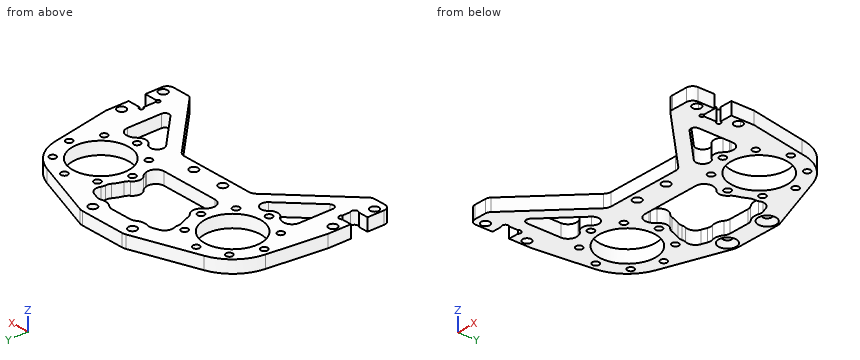
```python
from build123d import *

# Parameters (mm, degrees)
SKETCH_1_R          = 2.025
SKETCH_1_R_2        = 13.4
SKETCH_1_R_3        = 1.6
EXTRUDE_1_DEPTH     = 6
CHAMFER_1_SIZE      = 2.2
SKETCH_2_R          = 2.05
EXTRUDE_1_2_DEPTH   = 6
CUT_EXTRUDE_2_DEPTH = 7
SKETCH_4_R          = 1.525
CUT_EXTRUDE_3_DEPTH = 7
FILLET_1_R          = 3
CUT_EXTRUDE_6_DEPTH = 7
SKETCH_10_R         = 2.05
EXTRUDE_2_DEPTH     = 6
SKETCH_11_R         = 2.05
SKETCH_11_R_2       = 1
CUT_EXTRUDE_8_DEPTH = 7


with BuildPart() as part:
    # 草图1 → Extrude 1 (new body)
    with BuildSketch(Plane.XY):
        with BuildLine():
            Line((-43.507889071, -19.796198897), (-12.668545017, -30.71338069))
            ThreePointArc((-12.668545017, -30.71338069), (-11.846491746, -30.927824238), (-11, -31))
            Line((-11, -31), (11, -31))
            ThreePointArc((11, -31), (11.846491746, -30.927824238), (12.668545017, -30.71338069))
            Line((12.668545017, -30.71338069), (43.507889071, -19.796198897))
            ThreePointArc((43.507889071, -19.796198897), (57.5, 0), (43.507889071, 19.796198897))
            Line((43.507889071, 19.796198897), (12.668545017, 30.71338069))
            ThreePointArc((12.668545017, 30.71338069), (11.846491746, 30.927824238), (11, 31))
            Line((11, 31), (-11, 31))
            ThreePointArc((-11, 31), (-11.846491746, 30.927824238), (-12.668545017, 30.71338069))
            Line((-12.668545017, 30.71338069), (-43.507889071, 19.796198897))
            ThreePointArc((-43.507889071, 19.796198897), (-57.5, 0), (-43.507889071, -19.796198897))
        make_face()
        with Locations((-11, 26)):
            Circle(SKETCH_1_R, mode=Mode.SUBTRACT)
        with Locations((11, 26)):
            Circle(SKETCH_1_R, mode=Mode.SUBTRACT)
        with Locations((-36.5, 0)):
            Circle(SKETCH_1_R_2, mode=Mode.SUBTRACT)
        with Locations((-19, 0)):
            Circle(SKETCH_1_R_3, mode=Mode.SUBTRACT)
        with Locations((-24.125631329, -12.374368671)):
            Circle(SKETCH_1_R_3, mode=Mode.SUBTRACT)
        with Locations((-36.5, -17.5)):
            Circle(SKETCH_1_R_3, mode=Mode.SUBTRACT)
        with Locations((-48.874368671, -12.374368671)):
            Circle(SKETCH_1_R_3, mode=Mode.SUBTRACT)
        with Locations((-54, 0)):
            Circle(SKETCH_1_R_3, mode=Mode.SUBTRACT)
        with Locations((-48.874368671, 12.374368671)):
            Circle(SKETCH_1_R_3, mode=Mode.SUBTRACT)
        with Locations((-36.5, 17.5)):
            Circle(SKETCH_1_R_3, mode=Mode.SUBTRACT)
        with Locations((-24.125631329, 12.374368671)):
            Circle(SKETCH_1_R_3, mode=Mode.SUBTRACT)
        with Locations((36.5, 0)):
            Circle(SKETCH_1_R_2, mode=Mode.SUBTRACT)
        with Locations((19, 0)):
            Circle(SKETCH_1_R_3, mode=Mode.SUBTRACT)
        with Locations((24.125631329, 12.374368671)):
            Circle(SKETCH_1_R_3, mode=Mode.SUBTRACT)
        with Locations((36.5, 17.5)):
            Circle(SKETCH_1_R_3, mode=Mode.SUBTRACT)
        with Locations((48.874368671, 12.374368671)):
            Circle(SKETCH_1_R_3, mode=Mode.SUBTRACT)
        with Locations((54, 0)):
            Circle(SKETCH_1_R_3, mode=Mode.SUBTRACT)
        with Locations((48.874368671, -12.374368671)):
            Circle(SKETCH_1_R_3, mode=Mode.SUBTRACT)
        with Locations((36.5, -17.5)):
            Circle(SKETCH_1_R_3, mode=Mode.SUBTRACT)
        with Locations((24.125631329, -12.374368671)):
            Circle(SKETCH_1_R_3, mode=Mode.SUBTRACT)
        with Locations((-8, -20)):
            Circle(SKETCH_1_R, mode=Mode.SUBTRACT)
        with Locations((8, -20)):
            Circle(SKETCH_1_R, mode=Mode.SUBTRACT)
    extrude(amount=EXTRUDE_1_DEPTH)

    # 倒角1
    chamfer_1_edges = [part.edges().sort_by_distance(p)[0] for p in [
        (-13.025, 26, 0),
        (8.975, 26, 0),
    ]]
    chamfer(chamfer_1_edges, length=CHAMFER_1_SIZE)

    # 草圖2 → Extrude 1 2 (add)
    with BuildSketch(Plane(origin=(0, 0, 0), x_dir=(-1, 0, 0), z_dir=(0, 0, -1))):
        with BuildLine():
            Line((60.5, -55), (0, -55))
            Line((0, -55), (0, -31))
            Line((0, -31), (43.507889071, -19.796198897))
            ThreePointArc((43.507889071, -19.796198897), (54.311590133, -11.124174439), (57.363656278, 2.389110027))
            Line((57.363656278, 2.389110027), (60.5, -24.999999992))
            Line((60.5, -24.999999992), (60.5, -35.999999996))
            Line((60.5, -35.999999996), (53.5, -35.999999996))
            Line((53.5, -35.999999996), (53.5, -43.999999996))
            Line((53.5, -43.999999996), (60.5, -43.999999996))
            Line((60.5, -43.999999996), (60.5, -55))
        make_face()
        with Locations((57.5, -29.999999996)):
            Circle(SKETCH_2_R, mode=Mode.SUBTRACT)
        with Locations((57.5, -49.999999996)):
            Circle(SKETCH_2_R, mode=Mode.SUBTRACT)
    extrude_1_2 = extrude(amount=-EXTRUDE_1_2_DEPTH)

    # 草图3 → 切除-拉伸2 (cut, through all)
    with BuildSketch(Plane(origin=(0, 0, 0), x_dir=(-1, 0, 0), z_dir=(0, 0, -1))):
        with BuildLine():
            Line((50.5, -55), (20.671572875, -25.171572875))
            ThreePointArc((20.671572875, -25.171572875), (19.37387948, -24.30448187), (17.843145751, -24))
            Line((17.843145751, -24), (0, -24))
            Line((0, -24), (0, -55))
            Line((0, -55), (50.5, -55))
        make_face()
    cut_extrude_2 = extrude(amount=-CUT_EXTRUDE_2_DEPTH, mode=Mode.SUBTRACT)

    # 草图4 → 切除-拉伸3 (cut, through all)
    with BuildSketch(Plane(origin=(0, 0, 0), x_dir=(-1, 0, 0), z_dir=(0, 0, -1))):
        with Locations((54.578337841, -42.921662155)):
            Circle(SKETCH_4_R)
        with Locations((54.578337841, -37.078337837)):
            Circle(SKETCH_4_R)
    cut_extrude_3 = extrude(amount=-CUT_EXTRUDE_3_DEPTH, mode=Mode.SUBTRACT)

    # 鏡射2: Extrude 1 2, 切除-拉伸2, 切除-拉伸3 across plane
    add(extrude_1_2.mirror(Plane(origin=(0, 0, 0), x_dir=(0, 0, 1), z_dir=(1, 0, 0))))
    add(cut_extrude_2.mirror(Plane(origin=(0, 0, 0), x_dir=(0, 0, 1), z_dir=(1, 0, 0))), mode=Mode.SUBTRACT)
    add(cut_extrude_3.mirror(Plane(origin=(0, 0, 0), x_dir=(0, 0, 1), z_dir=(1, 0, 0))), mode=Mode.SUBTRACT)

    # 圆角1
    fillet_1_edges = [part.edges().sort_by_distance(p)[0] for p in [
        (-60.5, -55, 3),
        (-50.5, -55, 3),
        (60.5, -55, 3),
        (50.5, -55, 3),
    ]]
    fillet(fillet_1_edges, radius=FILLET_1_R)

    # 草图9 → 切除-拉伸6 (cut, through all)
    with BuildSketch(Plane(origin=(0, 0, 0), x_dir=(-1, 0, 0), z_dir=(0, 0, -1))):
        with BuildLine():
            Line((47.5, -38.686291501), (47.5, -22.433234274))
            ThreePointArc((47.5, -22.433234274), (45.870025586, -19.210971292), (42.308510638, -18.614811419))
            ThreePointArc((42.308510638, -18.614811419), (41.99756521, -18.709002559), (41.685093635, -18.798))
            ThreePointArc((41.685093635, -18.798), (40.572946608, -19.297500942), (39.662923531, -20.108814815))
            ThreePointArc((39.662923531, -20.108814815), (36.438317678, -21.599535985), (33.260020655, -20.01247564))
            ThreePointArc((33.260020655, -20.01247564), (28.487933079, -19.560886472), (28.337204639, -24.351923265))
            Line((28.337204639, -24.351923265), (44.085786438, -40.100505063))
            ThreePointArc((44.085786438, -40.100505063), (46.265366865, -40.534050566), (47.5, -38.686291501))
        make_face()
        with BuildLine():
            Line((-14.066765726, -11), (14.066765726, -11))
            ThreePointArc((14.066765726, -11), (17.289028708, -9.370025586), (17.885188581, -5.808510638))
            ThreePointArc((17.885188581, -5.808510638), (17.790997441, -5.49756521), (17.702, -5.185093635))
            ThreePointArc((17.702, -5.185093635), (17.202499058, -4.072946608), (16.391185185, -3.162923531))
            ThreePointArc((16.391185185, -3.162923531), (14.9, 0), (16.391185185, 3.162923531))
            ThreePointArc((16.391185185, 3.162923531), (17.202499058, 4.072946608), (17.702, 5.185093635))
            ThreePointArc((17.702, 5.185093635), (18.484349116, 7.462326931), (19.541391857, 9.625778403))
            ThreePointArc((19.541391857, 9.625778403), (19.974598058, 10.76538561), (20.044396006, 11.98255464))
            ThreePointArc((20.044396006, 11.98255464), (20.072251251, 12.990899237), (20.345463726, 13.961924305))
            ThreePointArc((20.345463726, 13.961924305), (20.315570737, 17.128932218), (17.992331346, 19.281463622))
            Line((17.992331346, 19.281463622), (15.321220814, 20.227041428))
            ThreePointArc((15.321220814, 20.227041428), (14.060319956, 20.455653517), (12.79183088, 20.273802126))
            ThreePointArc((12.79183088, 20.273802126), (9.984209905, 20.086610914), (7.4, 21.2))
            ThreePointArc((7.4, 21.2), (6.264911064, 21.794733192), (5, 22))
            Line((5, 22), (-5, 22))
            ThreePointArc((-5, 22), (-6.264911064, 21.794733192), (-7.4, 21.2))
            ThreePointArc((-7.4, 21.2), (-9.984209905, 20.086610914), (-12.79183088, 20.273802126))
            ThreePointArc((-12.79183088, 20.273802126), (-14.060319956, 20.455653517), (-15.321220814, 20.227041428))
            Line((-15.321220814, 20.227041428), (-17.992331346, 19.281463622))
            ThreePointArc((-17.992331346, 19.281463622), (-20.315570737, 17.128932218), (-20.345463726, 13.961924305))
            ThreePointArc((-20.345463726, 13.961924305), (-20.072251251, 12.990899237), (-20.044396006, 11.98255464))
            ThreePointArc((-20.044396006, 11.98255464), (-19.974598058, 10.76538561), (-19.541391857, 9.625778403))
            ThreePointArc((-19.541391857, 9.625778403), (-18.484349116, 7.462326931), (-17.702, 5.185093635))
            ThreePointArc((-17.702, 5.185093635), (-17.202499058, 4.072946608), (-16.391185185, 3.162923531))
            ThreePointArc((-16.391185185, 3.162923531), (-14.9, 0), (-16.391185185, -3.162923531))
            ThreePointArc((-16.391185185, -3.162923531), (-17.202499058, -4.072946608), (-17.702, -5.185093635))
            ThreePointArc((-17.702, -5.185093635), (-17.790997441, -5.49756521), (-17.885188581, -5.808510638))
            ThreePointArc((-17.885188581, -5.808510638), (-17.289028708, -9.370025586), (-14.066765726, -11))
        make_face()
        with BuildLine():
            Line((-28.337204639, -24.351923265), (-44.085786438, -40.100505063))
            ThreePointArc((-44.085786438, -40.100505063), (-46.265366865, -40.534050566), (-47.5, -38.686291501))
            Line((-47.5, -38.686291501), (-47.5, -22.433234274))
            ThreePointArc((-47.5, -22.433234274), (-45.870025586, -19.210971292), (-42.308510638, -18.614811419))
            ThreePointArc((-42.308510638, -18.614811419), (-41.99756521, -18.709002559), (-41.685093635, -18.798))
            ThreePointArc((-41.685093635, -18.798), (-40.572946608, -19.297500942), (-39.662923531, -20.108814815))
            ThreePointArc((-39.662923531, -20.108814815), (-36.438317678, -21.599535985), (-33.260020655, -20.01247564))
            ThreePointArc((-33.260020655, -20.01247564), (-28.487933079, -19.560886472), (-28.337204639, -24.351923265))
        make_face()
    extrude(amount=-CUT_EXTRUDE_6_DEPTH, mode=Mode.SUBTRACT)

    # 草图10 → 凸台-拉伸2 (add)
    with BuildSketch(Plane(origin=(0, 0, 0), x_dir=(-1, 0, 0), z_dir=(0, 0, -1))):
        with BuildLine():
            Line((-62.5, -43.999999996), (-57.656675683, -43.999999996))
            Line((-57.656675683, -43.999999996), (-55.5, -43.999999996))
            Line((-55.5, -43.999999996), (-55.5, -35.999999996))
            Line((-55.5, -35.999999996), (-57.5, -35.999999996))
            Line((-57.5, -35.999999996), (-62.5, -35.999999996))
            Line((-62.5, -35.999999996), (-62.5, -24.999999992))
            Line((-62.5, -24.999999992), (-57.363656278, 2.389110027))
            Line((-57.363656278, 2.389110027), (-51.742640687, -24.999999992))
            Line((-51.742640687, -24.999999992), (-51.742640687, -55))
            Line((-51.742640687, -55), (-59.5, -55))
            ThreePointArc((-59.5, -55), (-61.621320344, -54.121320344), (-62.5, -52))
            Line((-62.5, -52), (-62.5, -43.999999996))
        make_face()
        with Locations((-59.5, -29.999999996)):
            Circle(SKETCH_10_R, mode=Mode.SUBTRACT)
        with Locations((-59.5, -49.999999996)):
            Circle(SKETCH_10_R, mode=Mode.SUBTRACT)
    extrude(amount=-EXTRUDE_2_DEPTH)

    # 草图11 → 切除-拉伸8 (cut, through all)
    with BuildSketch(Plane.XY):
        with Locations((59.55, -29.999999996)):
            Circle(SKETCH_11_R)
        with Locations((59.55, -49.999999996)):
            Circle(SKETCH_11_R)
        with Locations((55.5, -35.999999996)):
            Circle(SKETCH_11_R_2)
        with Locations((55.5, -43.999999996)):
            Circle(SKETCH_11_R_2)
    extrude(amount=CUT_EXTRUDE_8_DEPTH, mode=Mode.SUBTRACT)


solid = part.part
```
Here's how the part is built. I have some questions about the finished solid (model axes, mm). Give positions to 0.01 mm unless a question says otherwise; leave off trailing zeros. Loops run counter-clockwise (first coordinate to the right, second up) from the corner with the lowest first, then second, coordinate; pieces in that order, holes last. Notation, with made-up numbers: M -39,28.25 L 18,28.25 A11 cw 18,39.25 Z; hole C 64.5,11 d6. An arc over 180 degrees is marked long. Use one line per item in the form item = value. Start each with the question number.
Q1. If we section it at D-D (z = 1): State how many separate pieces and enclosed holes the cut face has, then the cut area to 3 significant figures.
Q2. If we section it at B-B (x = 36.5): Write out the boundary of the cut face in (y, z).
Q3. Will these pins go through, and if not, where does the flat tip stop? pin 1 Ø3.5 at (x, y) = (-57.5, -30) entering from +Z; pin 2 Ø1 at (y, z) = (-21, 1.5) entering from +X; pin 3 Ø3 at (y, z) = (-39.5, 2) entering from -X; pin 4 Ø6.5 at (x, y) = (11, 26) entering from -Z (3 decimals).
Q4. I need wall thicknesses on line 1 along X through (y, z) = (-5.5, 1); line 2 along X through (y, z) = (-44.5, 1.5); line 3 along Y through (x, z) = (2, 3). Which ranges of each line are inside material? Lowest first, please.
Q5. If we section it at C-C (y = -30): Write out the boundary of the cut face in (x, z).
Q6. If we section it at A-A (x = 1.5): Write out the boundary of the cut face in (y, z).
Taken from the geometry:
q1.separate_pieces = 1
q1.enclosed_holes = 29
q1.area = 4,040 mm^2
q2.outline = M -41,0 L -32.51,0 L -32.51,6 L -41,6 Z; M -21.6,0 L -19.1,0 L -19.1,6 L -21.6,6 Z; M -15.9,0 L -13.4,0 L -13.4,6 L -15.9,6 Z; M 13.4,0 L 15.9,0 L 15.9,6 L 13.4,6 Z; M 19.1,0 L 22.28,0 L 22.28,6 L 19.1,6 Z
q3.pin_1 = through
q3.pin_2 = 61.84
q3.pin_3 = -53.5
q3.pin_4 = 0.975
q4.line_1 = -58.27 to -48.72, -24.28 to -17.79, 17.79 to 24.28, 48.72 to 58.84
q4.line_2 = -60.5 to -40, 40 to 54.63, 56.37 to 62.5
q4.line_3 = -24 to -11, 22 to 31
q5.outline = M -60.5,0 L -59.55,0 L -59.55,6 L -60.5,6 Z; M -55.45,0 L -47.5,0 L -47.5,6 L -55.45,6 Z; M -33.99,0 L -25.5,0 L -25.5,6 L -33.99,6 Z; M 25.5,0 L 33.99,0 L 33.99,6 L 25.5,6 Z; M 47.5,0 L 57.45,0 L 57.45,6 L 47.5,6 Z; M 61.6,0 L 62.5,0 L 62.5,6 L 61.6,6 Z
q6.outline = M -24,0 L -11,0 L -11,6 L -24,6 Z; M 22,0 L 31,0 L 31,6 L 22,6 Z
